from build123d import *

# Parameters (mm, degrees)
SKETCH1_W           = 40
SKETCH1_H           = 30
BOSS_EXTRUDE1_DEPTH = 8
SKETCH2_W           = 10
SKETCH2_H           = 30
BOSS_EXTRUDE2_DEPTH = 30
FILLET2_R           = 3
SKETCH3_R           = 2
CUT_EXTRUDE1_DEPTH  = 30
SKETCH4_R           = 2
CUT_EXTRUDE2_DEPTH  = 10
FILLET3_R           = 10


with BuildPart() as part:
    # Sketch1 → Boss-Extrude1 (new body)
    with BuildSketch(Plane(origin=(0, 0, 0), x_dir=(1, 0, 0), z_dir=(0, 1, 0))):
        Rectangle(SKETCH1_W, SKETCH1_H)
    extrude(amount=BOSS_EXTRUDE1_DEPTH)

    # Sketch2 → Boss-Extrude2 (add)
    with BuildSketch(Plane(origin=(0, 8, 0), x_dir=(1, 0, 0), z_dir=(0, 1, 0))):
        Rectangle(SKETCH2_W, SKETCH2_H)
    extrude(amount=BOSS_EXTRUDE2_DEPTH)

    # Fillet2
    fillet2_edges = [part.edges().sort_by_distance(p)[0] for p in [
        (5, 8, 0),
        (-5, 8, 0),
    ]]
    fillet(fillet2_edges, radius=FILLET2_R)

    # Sketch3 → Cut-Extrude1 (cut)
    with BuildSketch(Plane.XZ):
        with Locations(Location((-10, 9.706832571, 0), (0, 0, 270))):
            Circle(SKETCH3_R)
        with Locations(Location((10, 9.706832571, 0), (0, 0, 180))):
            Circle(SKETCH3_R)
        with Locations(Location((10, -9.706832571, 0), (0, 0, 270))):
            Circle(SKETCH3_R)
        with Locations((-10, -9.706832571)):
            Circle(SKETCH3_R)
    extrude(amount=-CUT_EXTRUDE1_DEPTH, mode=Mode.SUBTRACT)

    # Sketch4 → Cut-Extrude2 (cut)
    with BuildSketch(Plane(origin=(5, 0, 0), x_dir=(0, 0, -1), z_dir=(1, 0, 0))):
        with Locations((0, 26)):
            Circle(SKETCH4_R)
    extrude(amount=-CUT_EXTRUDE2_DEPTH, mode=Mode.SUBTRACT)

    # Fillet3
    fillet3_edges = [part.edges().sort_by_distance(p)[0] for p in [
        (0, 38, -15),
        (0, 38, 15),
    ]]
    fillet(fillet3_edges, radius=FILLET3_R)


solid = part.part
Verification items for the finished model (mm, model axes). A direction names the side the tool comes from. Coordinates: 2 decimals unless noted, no trailing zeros. Write each loop counter-clockwise with the first axis right and the second up, starting at its lowest first coordinate (ties: lowest second). Pieces come first, ordered by that corner, then holes. Notation, with made-up numbers: M -26,45 L -20,45 A30 ccw -20,69 Z; hole C -6,-17.5 d5. An arc over 180 degrees is marked long. Use CSV: the item, a comma, the result in double quotes.
Q1. Mould release check, pull along Z, two halves, no side actions. Record for faces 4 (the flat face through (0, 11, 15)), 5 (the cylindrical face through (-10.26, 3.944, -7.724)), 6 (the cylindrical face through (0.07, 35.15, -11.99)), 7 (the flat face through (-20, 4, 0)): pulls with the +Z half, pulls with the -Z half, needs draft (parallel to the pull), parting line crosses it, or undercut.
Computed values:
face 4,"pulls with the +Z half"
face 5,"undercut"
face 6,"pulls with the -Z half"
face 7,"needs draft"
Q2. Go/stop test with flat-tipped pins: P1, Ø3, axis at y = 26, z = 0, coming from the +X side; P2, Ø8, axis at x = -12, z = -11.5, coming from the -Y side; P3, Ø1.5, axis at x = 8.5, z = 10, coming from the +Y side; P4, Ø5, axis at y = 14, z = -7, coming from the -X side. Record where each tip stops, or that it passes through.
Computed values:
P1,"through"
P2,"y = 0"
P3,"y = 8.01"
P4,"x = -5"
Q3. Section check D-D, the plane y = 6. Enter the section's corners in (x, z), and give its area (3 significant figures).
Computed values:
outline,"M -20,-15 L 20,-15 L 20,15 L -20,15 Z; hole C -10,-9.71 d4; hole C -10,9.71 d4; hole C 10,-9.71 d4; hole C 10,9.71 d4"
area,"1,150 mm²"
Q4. Section check A-A, the plane x = -10. Enter the section's corners in (y, z), and give its area (3 significant figures).
Computed values:
outline,"M 0,-15 L 8,-15 L 8,-11.71 L 0,-11.71 Z; M 0,-7.71 L 8,-7.71 L 8,7.71 L 0,7.71 Z; M 0,11.71 L 8,11.71 L 8,15 L 0,15 Z"
area,"176 mm²"
Q5. Section check B-B, the plane y = 26. Enter the section's corners in (x, z), and give its area (3 significant figures).
Computed values:
outline,"M -5,-15 L 5,-15 L 5,-2 L -5,-2 Z; M -5,2 L 5,2 L 5,15 L -5,15 Z"
area,"260 mm²"
Q6. Set-up check for faces 1 (the flat face through (14, 8, 0)), 2 (the flat face through (0, 11, -15)), 3 (the flat face through (-14, 8, 0)): record each of +Z, -Z, +X, -X, +Y, -Y from which the full face is reachable in a straight line by a thin tool's end or side.
Computed values:
face 1,"+Z, -Z, +X, +Y"
face 2,"-Z, +X, -X, +Y, -Y"
face 3,"+Z, -Z, -X, +Y"
Q7. Thickness scan on line 1 along X through (y, z) = (3, -9); line 2 along Z through (x, y) = (-10, 4); line 3 along Y through (x, z) = (18, 5). Record the ranges inside material, lowest first. Write a range as [from, to].
Computed values:
line 1,"[-20, -11.87], [-8.13, 8.13], [11.87, 20]"
line 2,"[-15, -11.71], [-7.71, 7.71], [11.71, 15]"
line 3,"[0, 8]"
Q8. Section check C-C, the plane z = 0. Enter the section's corners in (x, y), and give its area (3 significant figures).
Computed values:
outline,"M -20,0 L 20,0 L 20,8 L 8,8 A3 cw 5,11 L 5,24 L -5,24 L -5,11 A3 cw -8,8 L -20,8 Z; M -5,28 L 5,28 L 5,38 L -5,38 Z"
area,"584 mm²"
